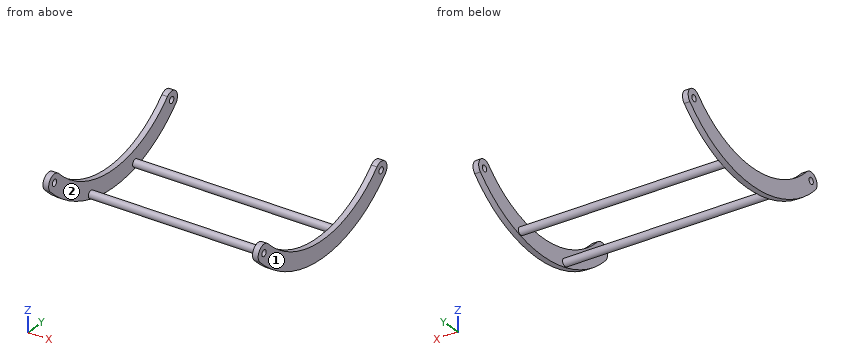
from build123d import *

# Parameters (mm, degrees)
BOSS_EXTRUDE1_DEPTH  = 3
SKETCH4_R            = 1.68
CUT_EXTRUDE1_DEPTH   = 54.466990195
SKETCH2_R            = 2
BOSS_EXTRUDE11_DEPTH = 108
SKETCH8_R            = 1.68
BOSS_EXTRUDE12_DEPTH = 3


with BuildPart() as part:
    # Sketch1 → Boss-Extrude1 (new body)
    with BuildSketch(Plane(origin=(0, 0, 0), x_dir=(0, 0, -1), z_dir=(1, 0, 0))):
        with BuildLine():
            ThreePointArc((-15.634588923, -40.698575462), (-15.635835692, -47.061289367), (-9.273122764, -47.06502941))
            ThreePointArc((-9.273122764, -47.06502941), (10.707664933, 1.119443717), (-9.273121767, 49.303917257))
            ThreePointArc((-9.273121767, 49.303917257), (-15.635834695, 49.300177346), (-15.634588058, 42.937463441))
            ThreePointArc((-15.634588058, 42.937463441), (1.687002572, 1.11944381), (-15.634588923, -40.698575462))
        make_face()
    extrude(amount=BOSS_EXTRUDE1_DEPTH)

    # Sketch4 → Cut-Extrude1 (cut, through all)
    with BuildSketch(Plane(origin=(3, 0, 0), x_dir=(0, 0, -1), z_dir=(1, 0, 0))):
        with Locations((-12.453854912, 46.120690349)):
            Circle(SKETCH4_R)
        with Locations((-12.453855844, -43.881802436)):
            Circle(SKETCH4_R)
    extrude(amount=-CUT_EXTRUDE1_DEPTH, mode=Mode.SUBTRACT)

    # Sketch2 → Boss-Extrude11 (add)
    with BuildSketch(Plane.ZY):
        with Locations(Location((-6.118587434, 18.157847035, 0), (0, 0, 180))):
            Circle(SKETCH2_R)
        with Locations(Location((-6.118587434, -15.875057848, 0), (0, 0, 180))):
            Circle(SKETCH2_R)
    extrude(amount=BOSS_EXTRUDE11_DEPTH)

    # Sketch8 → Boss-Extrude12 (add)
    with BuildSketch(Plane.ZY.offset(108)):
        with BuildLine():
            ThreePointArc((9.273121767, 49.303917257), (15.63708182, 49.301423495), (15.634588058, 42.937463441))
            ThreePointArc((15.634588058, 42.937463441), (-1.696602448, 1.11944381), (15.634588923, -40.698575462))
            ThreePointArc((15.634588923, -40.698575462), (15.637082818, -47.062535516), (9.273122764, -47.06502941))
            ThreePointArc((9.273122764, -47.06502941), (-10.696601757, 1.119443717), (9.273121767, 49.303917257))
        make_face()
        with Locations(Location((12.453854912, 46.120690349, 0), (0, 0, 180))):
            Circle(SKETCH8_R, mode=Mode.SUBTRACT)
        with Locations(Location((12.453855844, -43.881802436, 0), (0, 0, 180))):
            Circle(SKETCH8_R, mode=Mode.SUBTRACT)
    extrude(amount=BOSS_EXTRUDE12_DEPTH)


solid = part.part
Geometry check sheet. Reference: the model listing, model coordinates, mm. Face numbers are marked on the shaded views. Give positions to 0.01 mm unless a question says otherwise; leave off trailing zeros. Loops run counter-clockwise (first coordinate to the right, second up) from the corner with the lowest first, then second, coordinate; pieces in that order, holes last. Notation, with made-up numbers: M 38,82.25 L 74,82.25 A25 ccw 74,113.25 Z; hole C 8,38.5 d9. An arc over 180 degrees is marked long. Answer as a JSON object with one key per item and string values. Group by question number.
Item 1: Sectioned sample at B-B on y = -11. Record the boundary of the cut face in (x, z).
Item 2: Gauge pin test, flat ends, axial feed: pin 1 (2.5 mm diameter, centred on y = -43.88, z = 12.45, fed in from -X); pin 2 (2 mm diameter, centred on x = -39.5, z = -4, fed in from -Y); pin 3 (1.5 mm diameter, centred on x = -30.5, z = -7.5, fed in from -Y); pin 4 (8 mm diameter, centred on x = -93.5, y = -11.5, fed in from +Z). Record the tip position at first contact, or that the pin passes through.
Item 3: Material ranges on L1, parallel to X at y = -22, z = -6, recorded low to high.
Item 4: Mould release check, pull along Y, two halves, no side actions. Record for the marked faces 1 and 2: pulls with the +Y half, pulls with the -Y half, needs draft (parallel to the pull), parting line crosses it, or undercut.
Item 5: Sectioned sample at C-C on x = -53. Record the boundary of the cut face in (y, z).
Item 6: Sectioned sample at D-D on y = -28.5. Record the boundary of the cut face in (x, z).
Item 7: Sectioned sample at A-A on z = 3.5. Record the boundary of the cut face in (x, y).
Findings below:
{
 "1": {"outline": "M -111,-9.61 L -108,-9.61 L -108,-0.44 L -111,-0.44 Z; M 0,-9.62 L 3,-9.62 L 3,-0.43 L 0,-0.43 Z"},
 "2": {"pin 1": "through", "pin 2": "y = -17.53", "pin 3": "y = -17.77", "pin 4": "z = -4.15"},
 "3": {"L1": "-111 to -108, 0 to 3"},
 "4": {"face 1": "needs draft", "face 2": "undercut"},
 "5": {"outline": "C -15.88,-6.12 d4; C 18.16,-6.12 d4"},
 "6": {"outline": "M -111,-3.92 L -108,-3.92 L -108,6.26 L -111,6.26 Z; M 0,-3.93 L 3,-3.93 L 3,6.26 L 0,6.26 Z"},
 "7": {"outline": "M -111,-40.5 L -108,-40.5 L -108,-23.12 L -111,-23.12 Z; M -111,25.36 L -108,25.36 L -108,42.74 L -111,42.74 Z; M 0,-40.51 L 3,-40.51 L 3,-23.1 L 0,-23.1 Z; M 0,25.34 L 3,25.34 L 3,42.75 L 0,42.75 Z"}
}
